Read the model definition and answer for the solid it produces. Units are mm, in the model's axes. A direction names the side the tool comes from. Round coordinates to 2 decimals unless told otherwise and drop trailing zeros. Write each loop counter-clockwise with the first axis right and the second up, starting at its lowest first coordinate (ties: lowest second). Pieces come first, ordered by that corner, then holes. Notation, with made-up numbers: (80, 17.5) -> (92, 17.5) arc R18 ccw to (92, 50.5) -> close; hole circle Ø3 at (47.25, 7.5). An arc over 180 degrees is marked (long way). Return JSON: item names as keys, results as strings. Group by question number.
(1) The mould has two halves that part along Y. Classify faces 5 (the flat face through (27, -49, -2)), 6 (the flat face through (164, 4, -2)), 7 (the flat face through (171, -47, -2)), 8 (the flat face through (21, -4, -3)): released by +Y, released by -Y, zero draft, split by the parting line, or undercut.
(2) Given pin 1 (1.2 mm diameter, centred on y = -49.5, z = -2, fed in from +X); pin 2 (5 mm diameter, centred on x = 173.75, y = -15.65, fed in from -Z); pin 3 (2 mm diameter, centred on x = 139, z = -2, fed in from +Y); pin 4 (1.2 mm diameter, centred on x = 29, z = -2.5, fed in from -Y), each flat-ended and moving along its own axis, determine where each tip first touches the part or whether it passes through.
(3) A cutting plane is placed at C-C on x = 119.5. Give the vertices of the cut face in (y, z).
(4) A cutting plane is placed at B-B on x = 143.75. Give the vertices of the cut face in (y, z).
(5) For faces 1 (the flat face through (159, -39, -2)), 2 (the flat face through (10, -47, -2)), 3 (the flat face through (141, -49, -2)), 4 (the flat face through (174, 0, -2)), determine the directions among +Z, -Z, +X, -X, +Y, -Y from which every point of the face is accessible in a straight line to the end or side of a thin tool.
(6) A cutting plane is placed at D-D on z = -2. State how many separate pieces and enclosed holes the cut face has, then the cut area to 3 significant figures.
(7) A cutting plane is placed at A-A on y = -45. Give the vertices of the cut face in (x, z), then the cut area to 3 significant figures.
(8) Straight lines are drawn through the part: line 1 (X direction, y = -14, z = -1.25); line 2 (X direction, y = -41.4, z = -2); line 3 (Y direction, x = 173.75, z = -3.05). For each, find the intervals that lie inside material, in ascending order.
```python
from build123d import *

# Parameters (mm, degrees)
SKETCH_1_R             = 1.6
SKETCH_1_R_2           = 5.5
SKETCH_1_R_3           = 1.5
SKETCH_1_W             = 12.5
SKETCH_1_H             = 12.5
SKETCH_1_W_2           = 20
SKETCH_1_H_2           = 12
SM_BASE_FLANGE_1_DEPTH = 4
SKETCH_6_R             = 1
CUT_EXTRUDE_1_DEPTH    = 10
SKETCH_7_R             = 1
CUT_EXTRUDE_2_DEPTH    = 10


# Sheet-metal steps are written as plain solids
with BuildPart() as part:
    # Sketch 1 → Базовая кромка1 (new body)
    with BuildSketch(Plane.XY):
        with BuildLine():
            Line((0, 0), (12, 0))
            Line((12, 0), (12, 4))
            Line((12, 4), (20, 4))
            Line((20, 4), (20, 0))
            Line((20, 0), (18, 0))
            Line((18, 0), (18, -4))
            Line((18, -4), (26, -4))
            Line((26, -4), (26, 0))
            Line((26, 0), (24, 0))
            Line((24, 0), (24, 4))
            Line((24, 4), (32, 4))
            Line((32, 4), (32, 0))
            Line((32, 0), (50, 0))
            Line((50, 0), (50, -29))
            ThreePointArc((50, -29), (51.171572875, -31.828427125), (54, -33))
            Line((54, -33), (126, -33))
            ThreePointArc((126, -33), (128.828427125, -31.828427125), (130, -29))
            Line((130, -29), (130, 0))
            Line((130, 0), (148, 0))
            Line((148, 0), (148, 4))
            Line((148, 4), (156, 4))
            Line((156, 4), (156, 0))
            Line((156, 0), (154, 0))
            Line((154, 0), (154, -4))
            Line((154, -4), (162, -4))
            Line((162, -4), (162, 0))
            Line((162, 0), (160, 0))
            Line((160, 0), (160, 4))
            Line((160, 4), (168, 4))
            Line((168, 4), (168, 0))
            Line((168, 0), (180, 0))
            Line((180, 0), (180, -47))
            Line((180, -47), (161, -47))
            Line((161, -47), (161, -51))
            Line((161, -51), (153, -51))
            Line((153, -51), (153, -47))
            Line((153, -47), (155, -47))
            Line((155, -47), (155, -43))
            Line((155, -43), (147, -43))
            Line((147, -43), (147, -47))
            Line((147, -47), (149, -47))
            Line((149, -47), (149, -51))
            Line((149, -51), (141, -51))
            Line((141, -51), (141, -47))
            Line((141, -47), (90, -47))
            Line((90, -47), (39, -47))
            Line((39, -47), (39, -51))
            Line((39, -51), (31, -51))
            Line((31, -51), (31, -47))
            Line((31, -47), (33, -47))
            Line((33, -47), (33, -43))
            Line((33, -43), (25, -43))
            Line((25, -43), (25, -47))
            Line((25, -47), (27, -47))
            Line((27, -47), (27, -51))
            Line((27, -51), (19, -51))
            Line((19, -51), (19, -47))
            Line((19, -47), (0, -47))
            Line((0, -47), (0, 0))
        make_face()
        with Locations((143.75, -15.647183543)):
            Circle(SKETCH_1_R, mode=Mode.SUBTRACT)
        with Locations((173.75, -15.647183543)):
            Circle(SKETCH_1_R, mode=Mode.SUBTRACT)
        with Locations((143.75, -33)):
            Circle(SKETCH_1_R, mode=Mode.SUBTRACT)
        with Locations((173.75, -33)):
            Circle(SKETCH_1_R, mode=Mode.SUBTRACT)
        with Locations((21.194446521, -33)):
            Circle(SKETCH_1_R_2, mode=Mode.SUBTRACT)
        with Locations((90, -37)):
            Circle(SKETCH_1_R_3, mode=Mode.SUBTRACT)
        with Locations((54, -37)):
            Circle(SKETCH_1_R_3, mode=Mode.SUBTRACT)
        with Locations((126, -37)):
            Circle(SKETCH_1_R_3, mode=Mode.SUBTRACT)
        with Locations((12.694446521, -15.647183543)):
            Circle(SKETCH_1_R_3, mode=Mode.SUBTRACT)
        with Locations((29.694446521, -15.647183543)):
            Circle(SKETCH_1_R_3, mode=Mode.SUBTRACT)
        with Locations((158.75, -15.647183543)):
            Rectangle(SKETCH_1_W, SKETCH_1_H, mode=Mode.SUBTRACT)
        with Locations((158.75, -33)):
            Rectangle(SKETCH_1_W_2, SKETCH_1_H_2, mode=Mode.SUBTRACT)
        with BuildLine():
            Line((15.944446521, -12.147183543), (26.444446521, -12.147183543))
            ThreePointArc((26.444446521, -12.147183543), (27.151553303, -12.440076762), (27.444446521, -13.147183543))
            Line((27.444446521, -13.147183543), (27.444446521, -18.147183543))
            ThreePointArc((27.444446521, -18.147183543), (27.151553303, -18.854290324), (26.444446521, -19.147183543))
            Line((26.444446521, -19.147183543), (15.944446521, -19.147183543))
            ThreePointArc((15.944446521, -19.147183543), (15.23733974, -18.854290324), (14.944446521, -18.147183543))
            Line((14.944446521, -18.147183543), (14.944446521, -13.147183543))
            ThreePointArc((14.944446521, -13.147183543), (15.23733974, -12.440076762), (15.944446521, -12.147183543))
        make_face(mode=Mode.SUBTRACT)
    extrude(amount=-SM_BASE_FLANGE_1_DEPTH)

    # Эскиз6 → Вырез-Вытянуть1 (cut)
    with BuildSketch(Plane(origin=(0, 4, 0), x_dir=(1, 0, 0), z_dir=(0, 1, 0))):
        with Locations(Location((22, 2, 0), (0, 0, 180))):
            Circle(SKETCH_6_R)
        with Locations(Location((158, 2, 0), (0, 0, 180))):
            Circle(SKETCH_6_R)
    extrude(amount=-CUT_EXTRUDE_1_DEPTH, mode=Mode.SUBTRACT)

    # Эскиз7 → Вырез-Вытянуть2 (cut)
    with BuildSketch(Plane.XZ.offset(51)):
        with Locations(Location((29, -2, 0), (0, 0, 270))):
            Circle(SKETCH_7_R)
        with Locations(Location((151, -2, 0), (0, 0, 270))):
            Circle(SKETCH_7_R)
    extrude(amount=-CUT_EXTRUDE_2_DEPTH, mode=Mode.SUBTRACT)


solid = part.part
```
Checks:
{
 "1": {"face 5": "zero draft", "face 6": "released by +Y", "face 7": "released by -Y", "face 8": "undercut"},
 "2": {"pin 1": "stops at x = 161", "pin 2": "stops at z = -4", "pin 3": "stops at y = 0", "pin 4": "stops at y = -43"},
 "3": {"outline": "(-47, -4) -> (-33, -4) -> (-33, 0) -> (-47, 0) -> close"},
 "4": {"outline": "(-51, -4) -> (-34.6, -4) -> (-34.6, 0) -> (-51, 0) -> close; (-31.4, -4) -> (-17.25, -4) -> (-17.25, 0) -> (-31.4, 0) -> close; (-14.05, -4) -> (0, -4) -> (0, 0) -> (-14.05, 0) -> close"},
 "5": {"face 1": "+Z, -Z", "face 2": "+Z, -Z, -X, -Y", "face 3": "+Z, -Z, -Y", "face 4": "+Z, -Z, +X, +Y"},
 "6": {"separate pieces": "1", "enclosed holes": "13", "area": "5,290 mm^2"},
 "7": {"outline": "(0, -4) -> (25, -4) -> (25, 0) -> (0, 0) -> close; (33, -4) -> (147, -4) -> (147, 0) -> (33, 0) -> close; (155, -4) -> (180, -4) -> (180, 0) -> (155, 0) -> close", "area": "656 mm^2"},
 "8": {"line 1": "x = 0 to 14.94, 27.44 to 50, 130 to 152.5, 165 to 180", "line 2": "x = 0 to 28, 30 to 150, 152 to 180", "line 3": "y = -47 to -34.6, -31.4 to -17.25, -14.05 to 0"}
}
